Could you check a few things on this model? Use its own coordinates, in mm. Face numbers are marked on the shaded views. A direction names the side the tool comes from. Coordinates: 2 decimals unless noted, no trailing zeros. Order: outer loops, then holes, each group sorted by start corner. A loop starts at its lowest first (then second) coordinate and runs counter-clockwise, first axis right, second up. Notation, with made-up numbers: (14, 54.25) -> (57, 54.25) arc R25 ccw to (57, 72.25) -> close; hole circle Ø6 at (24.5, -28). An arc over 180 degrees is marked (long way). Use a Markdown table: item, result. Add a question column.
1) If I drill on L1, parallel to Y at x = 7, z = 15.5; L2, parallel to X at y = 84, z = 0.5; L3, parallel to X at y = 157, z = 2.5, over which ranges is the centre line in solid material (lowest first)? Write a range as [from, to].
2) If we section it at C-C (x = 0): Write out the boundary of the cut face in (y, z), plus the area to 3 significant figures.
3) If we section it at A-A (x = -13): Write out the boundary of the cut face in (y, z) (3 decimals), plus the area to 3 significant figures.
4) If we section it at B-B (y = 177): Write out the boundary of the cut face in (x, z), plus the area to 3 significant figures.
5) Which directions (+Z, -Z, +X, -X, +Y, -Y) give clear straight access to the entire face, cutting with the end or side of a thin tool? Please do the marked faces 1 and 2.
6) If we section it at D-D (z = -22): Write out the boundary of the cut face in (x, y).
7) Will these pins go through, and if not, where does the flat tip stop? pin 1 Ø6 at (x, z) = (27.5, 5.5) entering from -Y; pin 2 Ø6 at (x, y) = (19.5, 21) entering from +Z.
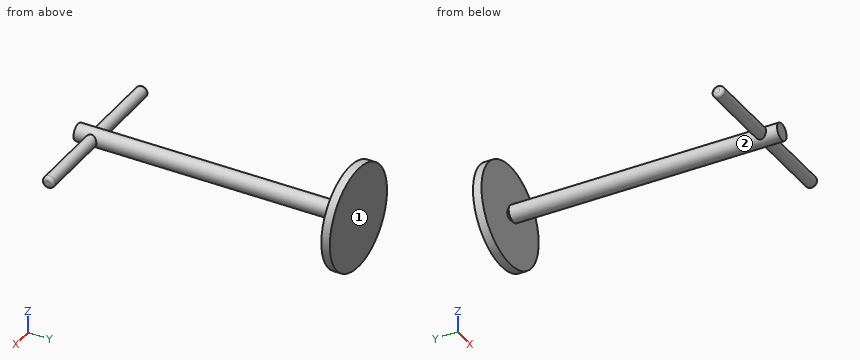
```python
from build123d import *

# Parameters (mm, degrees)
SKETCH1_R           = 6.35
BOSS_EXTRUDE1_DEPTH = 203.2
CHAMFER1_SIZE       = 2.54
SKETCH3_R           = 38.1
BOSS_EXTRUDE2_DEPTH = 6.35
SKETCH4_R           = 4.445
BOSS_EXTRUDE3_DEPTH = 63.5
FILLET2_R           = 2.54


with BuildPart() as part:
    # Sketch1 → Boss-Extrude1 (new body)
    with BuildSketch(Plane(origin=(0, 0, 0), x_dir=(1, 0, 0), z_dir=(0, 1, 0))):
        with Locations(Location((0, 0, 0), (0, 0, 270))):
            Circle(SKETCH1_R)
    extrude(amount=BOSS_EXTRUDE1_DEPTH)

    # Chamfer1
    chamfer1_edges = [part.edges().sort_by_distance(p)[0] for p in [
        (0, 203.2, -6.35),
    ]]
    chamfer(chamfer1_edges, length=CHAMFER1_SIZE)

    # Sketch3 → Boss-Extrude2 (add)
    with BuildSketch(Plane(origin=(0, 203.2, 0), x_dir=(1, 0, 0), z_dir=(0, 1, 0))):
        with Locations(Location((0, 0, 0), (0, 0, 270))):
            Circle(SKETCH3_R)
    extrude(amount=BOSS_EXTRUDE2_DEPTH)

    # Sketch4 → Boss-Extrude3 (add, symmetric)
    with BuildSketch(Plane(origin=(0, 0, 0), x_dir=(0, 0, -1), z_dir=(1, 0, 0))):
        with Locations(Location((0, 12.7, 0), (0, 0, 180))):
            Circle(SKETCH4_R)
    extrude(amount=BOSS_EXTRUDE3_DEPTH, both=True)

    # Fillet2
    fillet2_edges = [part.edges().sort_by_distance(p)[0] for p in [
        (-63.5, 12.7, -4.445),
        (63.5, 12.7, -4.445),
    ]]
    fillet(fillet2_edges, radius=FILLET2_R)


solid = part.part
```
Answer sheet:
| question | item | result |
|---|---|---|
| 1 | L1 | [203.2, 209.55] |
| 1 | L2 | [-6.33, 6.33] |
| 1 | L3 | [-5.84, 5.84] |
| 2 | outline | (0, -6.35) -> (200.66, -6.35) -> (203.2, -3.81) -> (203.2, -38.1) -> (209.55, -38.1) -> (209.55, 38.1) -> (203.2, 38.1) -> (203.2, 3.81) -> (200.66, 6.35) -> (0, 6.35) -> close |
| 2 | area | 3,060 mm2 |
| 3 | outline | circle Ø8.89 at (12.7, 0); (203.2, -35.814) -> (209.55, -35.814) -> (209.55, 35.814) -> (203.2, 35.814) -> close |
| 3 | area | 517 mm2 |
| 4 | outline | circle Ø12.7 at (0, 0) |
| 4 | area | 127 mm2 |
| 5 | face 1 | +Z, -Z, +X, -X, +Y |
| 5 | face 2 | none |
| 6 | outline | (-31.11, 203.2) -> (31.11, 203.2) -> (31.11, 209.55) -> (-31.11, 209.55) -> close |
| 7 | pin 1 | y = 9.02 |
| 7 | pin 2 | through |
